Source: CAD feature listing. Evaluate the final solid. Frame: model axes, mm. A direction names the side the tool comes from. Round coordinates to 2 decimals unless told otherwise and drop trailing zeros. Loops run counter-clockwise (first coordinate to the right, second up) from the corner with the lowest first, then second, coordinate; pieces in that order, holes last. Notation, with made-up numbers: (54, 37.5) - (79, 37.5) arc R25 cw to (79, 76.5) - close; hole circle Ø8 at (73, 88.25). An arc over 180 degrees is marked (long way). One line per question, with ' | ' between items.
from build123d import *

# Parameters (mm, degrees)
F1_DEPTH = 254
F2_R     = 10.393526
F3_DEPTH = 25.4


with BuildPart() as f1:
    # F0 (on Right) → F1 (new body)
    with BuildSketch(Plane.YZ):
        Polygon((73.321618, 0), (68.32242, 46.414401), (0, 46.414401), (0, 0), align=None)
    extrude(amount=F1_DEPTH)

    # F2 (on face) → F3 (join)
    with BuildSketch(Plane.XZ):
        with Locations((140.782937, 27.210025)):
            Circle(F2_R)
    extrude(amount=F3_DEPTH)


solid = f1.part
1. Access query for faces 1 (the flat face through (141, -25.4, 27)), 2 (the cylindrical face through (132.53, -12.52, 20.89)). Directions: +Z, -Z, +X, -X, +Y, -Y. A direction counts if a zero-diameter tool reaches every point of the face in a straight line with its end or side. Return the directions, or none.
Worked out:
face 1: +Z, -Z, +X, -X, -Y | face 2: -Y
2. Section query C-C, the plane z = 42. Return loops of the section in (x, y), plus the area to 3 significant figures.
Worked out:
outline: (0, 0) - (254, 0) - (254, 68.8) - (0, 68.8) - close | area: 17,500 mm2
3. Material intervals for probe 1 along Y at (x, z) = (236.5, 8.5); probe 2 along Y at (x, z) = (43, 42.5), sorted ascending.
Worked out:
probe 1: y = 0 to 72.41 | probe 2: y = 0 to 68.74
4. Contact query for flat-ended pins moving along their axis: P1, Ø8, axis at x = 179, z = 35.5, coming from the +Y side; P2, Ø10, axis at x = 56, z = 34.5, coming from the -Y side; P3, Ø4, axis at x = 202, z = 22, coming from the +Y side. Output: stop coordinate, or through.
Worked out:
P1: stops at y = 69.93 | P2: stops at y = 0 | P3: stops at y = 71.17
5. Section query B-B, the plane x = 200.5. Return loops of the section in (y, z), plus the area to 3 significant figures.
Worked out:
outline: (0, 0) - (73.32, 0) - (68.32, 46.41) - (0, 46.41) - close | area: 3,290 mm2
6. Section query A-A, the plane z = 20. Return loops of the section in (x, y), plus the area to 3 significant figures.
Worked out:
outline: (0, 0) - (133.3, 0) - (133.3, -25.4) - (148.27, -25.4) - (148.27, 0) - (254, 0) - (254, 71.17) - (0, 71.17) - close | area: 18,500 mm2
